Verification items for this drawing (mm, ordinates from the low corner). A direction names the side the tool comes from. Give positions to 0.01 mm unless a question says otherwise; leave off trailing zeros. Loops run counter-clockwise (first coordinate to the right, second up) from the corner with the lowest first, then second, coordinate; pieces in that order, holes last. Notation, with made-up numbers: M -20.5,80.25 L 23.5,80.25 A18 cw 23.5,104.25 Z; hole C 0,-23 d11. An arc over 180 degrees is marked long. Use a Markdown table: item, result.
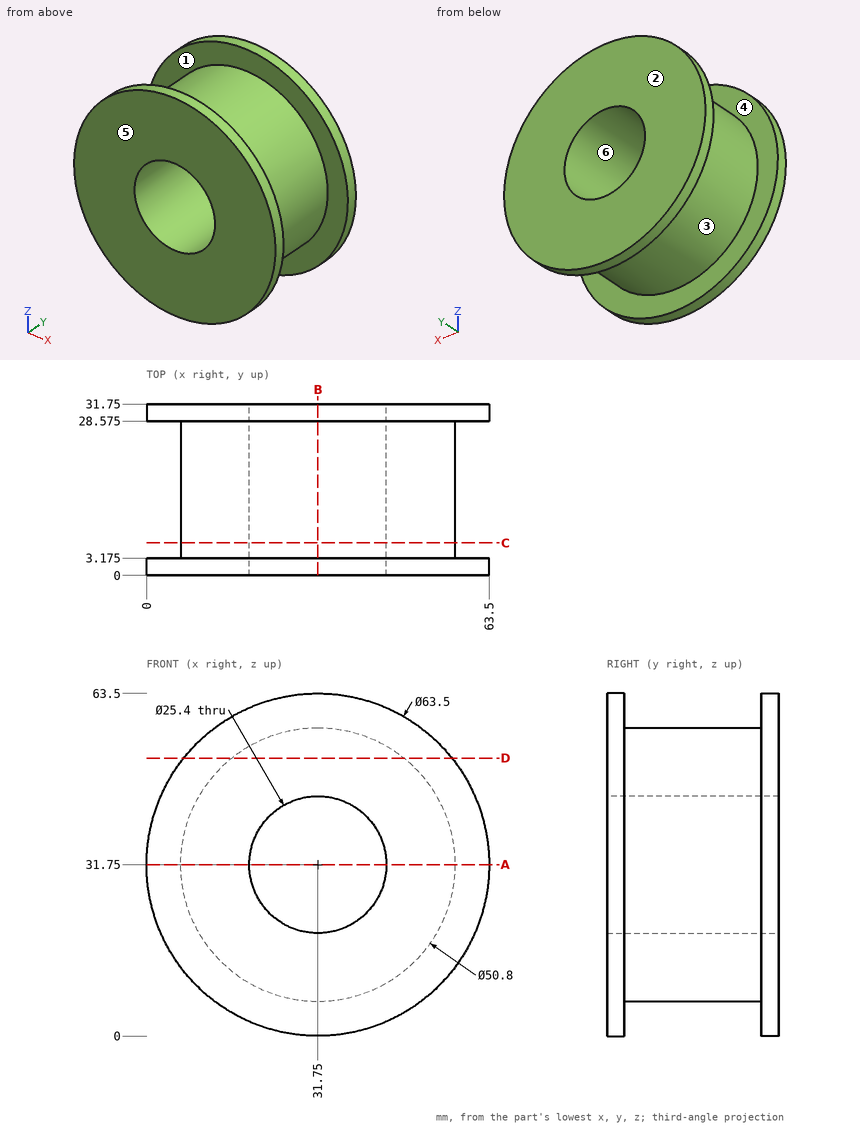
(1) Gauge pin test, flat ends, axial feed: P1, Ø1.5, axis at x = 53, y = 9.5, coming from the +Z side; P2, Ø2, axis at x = 27.5, y = 24.5, coming from the -Z side; P3, Ø6, axis at x = 46, z = 44.5, coming from the -Y side; P4, Ø4, axis at y = 19, z = 17, coming from the +X side. Record the tip position at first contact, or that the pin passes through.
Results below:
| item | result |
|---|---|
| P1 | z = 46.75 |
| P2 | z = 6.56 |
| P3 | y = 0 |
| P4 | x = 53.72 |
(2) Draft check along Y on the marked faces 3, 4, 5 and 6. Enter one of: +Y half, -Y half, draft (parallel to the pull), parting line (faces both ways), or undercut.
Results below:
| item | result |
|---|---|
| face 3 | undercut |
| face 4 | undercut |
| face 5 | -Y half |
| face 6 | draft |
(3) Cross-section at B-B on x = 31.75. Record the cut outline in (y, z) (3 decimals), then the cut area to 3 significant figures.
Results below:
| item | result |
|---|---|
| outline | M 0,0 L 3.175,0 L 3.175,6.35 L 28.575,6.35 L 28.575,0 L 31.75,0 L 31.75,19.05 L 0,19.05 Z; M 0,44.45 L 31.75,44.45 L 31.75,63.5 L 28.575,63.5 L 28.575,57.15 L 3.175,57.15 L 3.175,63.5 L 0,63.5 Z |
| area | 887 mm^2 |
(4) Cross-section at D-D on z = 51.5. Record the cut outline in (x, y) (3 decimals).
Results below:
| item | result |
|---|---|
| outline | M 6.89,0 L 56.61,0 L 56.61,3.175 L 47.722,3.175 L 47.722,28.575 L 56.61,28.575 L 56.61,31.75 L 6.89,31.75 L 6.89,28.575 L 15.778,28.575 L 15.778,3.175 L 6.89,3.175 Z |
(5) Set-up check for the marked faces 1 and 2: record each of +Z, -Z, +X, -X, +Y, -Y from which the full face is reachable in a straight line by a thin tool's end or side.
Results below:
| item | result |
|---|---|
| face 1 | none |
| face 2 | +Z, -Z, +X, -X, +Y |
(6) Cross-section at A-A on z = 31.75. Record the cut outline in (x, y) (3 decimals), then the cut area to 3 significant figures.
Results below:
| item | result |
|---|---|
| outline | M 0,0 L 19.05,0 L 19.05,31.75 L 0,31.75 L 0,28.575 L 6.35,28.575 L 6.35,3.175 L 0,3.175 Z; M 44.45,0 L 63.5,0 L 63.5,3.175 L 57.15,3.175 L 57.15,28.575 L 63.5,28.575 L 63.5,31.75 L 44.45,31.75 Z |
| area | 887 mm^2 |
(7) Material ranges on line 1 (Y direction, x = 58.5, z = 39) (3 decimals); line 2 (X direction, y = 8, z = 31.75); line 3 (Z direction, x = 31, y = 16), recorded low to high.
Results below:
| item | result |
|---|---|
| line 1 | 0 to 3.175, 28.575 to 31.75 |
| line 2 | 6.35 to 19.05, 44.45 to 57.15 |
| line 3 | 6.36 to 19.07, 44.43 to 57.14 |
(8) Cross-section at C-C on y = 6. Record the cut outline in (x, z).
Results below:
| item | result |
|---|---|
| outline | C 31.75,31.75 d50.8; hole C 31.75,31.75 d25.4 |
